Can you work these out from the model? Positions are in its coordinate system, mm. Face numbers are marked on the shaded views. A direction names the side the tool comes from. Give positions to 0.01 mm unless a question says otherwise; leave off trailing zeros. Write each loop counter-clockwise with the first axis right and the second up, starting at its lowest first coordinate (ties: lowest second). Pieces come first, ordered by that corner, then holes. Notation, with made-up numbers: M -26,-4 L 27,-4 A21 cw 27,28 Z; hole C 76,39 d3. An arc over 180 degrees is marked long. Use CSV: the item, a comma, the result in double quotes. Start each with the question number.
from build123d import *

# Parameters (mm, degrees)
F1_DEPTH  = 50.8
F3_DEPTH  = 16.51
F6_DEPTH  = 12.7
F4_R      = 7.62
F7_DEPTH  = 19.05
F8_R      = 6.35
F9_DEPTH  = 70.358
F10_R     = 7.62
F11_DEPTH = 17.018


with BuildPart() as f1:
    # F0 (on Front) → F1 (new body)
    with BuildSketch(Plane.XZ):
        Polygon((-5.651368, 9.435547), (-10.997107, -0.176455), (-5.345739, -9.612001), (5.651368, -9.435547), (10.997107, 0.176455), (5.345739, 9.612001), align=None)
    extrude(amount=F1_DEPTH)

    # F2 (on Right) → F3 (join)
    with BuildSketch(Plane.YZ):
        Polygon((-19.900739, 9.525), (-30.899261, 9.525), (-36.398523, 0), (-30.899261, -9.525), (-19.900739, -9.525), (-14.401477, 0), align=None)
    extrude(amount=-F3_DEPTH)

    # F5 (on face) → F6 (join)
    with BuildSketch(Plane.XZ.offset(50.8)):
        Polygon((-4.356068, 11.679071), (-12.292406, 2.06707), (-7.936338, -9.612001), (4.356068, -11.679071), (12.292406, -2.06707), (7.936338, 9.612001), align=None)
    extrude(amount=F6_DEPTH)

    # F4 (on face) → F7 (join)
    with BuildSketch(Plane(origin=(0, 0, 0), x_dir=(-1, 0, 0), z_dir=(0, 1, 0))):
        Circle(F4_R)
    extrude(amount=F7_DEPTH)

    # F8 (on face) → F9 (cut)
    with BuildSketch(Plane(origin=(0, 19.05, 0), x_dir=(-1, 0, 0), z_dir=(0, 1, 0))):
        Circle(F8_R)
    extrude(amount=-F9_DEPTH, mode=Mode.SUBTRACT)

    # F10 (on face) → F11 (cut)
    with BuildSketch(Plane(origin=(-16.51, 0, 0), x_dir=(0, -1, 0), z_dir=(-1, 0, 0))):
        with Locations((25.4, 0)):
            Circle(F10_R)
    extrude(amount=-F11_DEPTH, mode=Mode.SUBTRACT)


solid = f1.part
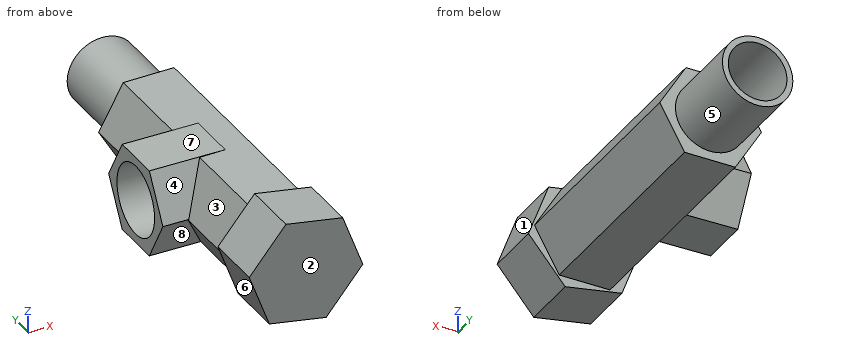
(1) Please list where these lines run through material, in increasing order: L1, parallel to Y at x = -10.75, z = 0; L2, parallel to Z at x = 0, y = -4.5; L3, parallel to Z at x = -9.5, y = -25.4 (3 decimals). Write a range as [from, to].
(2) I want a section at A-A (y = 4.5). Write out the boundary of the cut face in (x, z).
(3) Thinking about a two-plate mould opening in Y: for the marked faces 1, 2 and 3, which applies, released by +Y, released by -Y, zero draft, split by the parting line, or undercut?
(4) Which directions (+Z, -Z, +X, -X, +Y, -Y) give clear straight access to the entire face, cutting with the end or side of a thin tool? Please do the marked faces 4, 5, 6, 7 and 8.
(5) Will these pins go through, and if not, where does the flat tip stop? pin 1 Ø7 at (x, z) = (-1.5, 5.5) entering from +Y; pin 2 Ø10 at (x, y) = (-10.5, -33.5) entering from -Z (3 decimals); pin 3 Ø1.5 at (x, y) = (-3.5, 8.5) entering from -Z; pin 4 Ø8 at (y, z) = (-45, 9) entering from +X.
(6) I want a section at D-D (y = -25.4). Write out the boundary of the cut face in (x, z) (3 decimals), and give its area (3 significant figures).
(7) I want a section at C-C (x = -3.25). Write out the boundary of the cut face in (y, z) (3 decimals), and give its area (3 significant figures).
(8) I want a section at B-B (z = 3.5). Write out the boundary of the cut face in (x, y), and give its area (3 significant figures).
Geometry results:
1,L1,"y = [-63.5, -33.02], [-17.78, 0]"
1,L2,"z = [-9.53, -6.35], [6.35, 9.53]"
1,L3,"z = [-9.525, -7.62], [7.62, 9.525]"
2,outline,"C 0,0 d15.24; hole C 0,0 d12.7"
3,face 1,"zero draft"
3,face 2,"released by -Y"
3,face 3,"undercut"
4,face 4,"+Z, -X"
4,face 5,"+Y"
4,face 6,"-Z, -X, -Y"
4,face 7,"+Z, -X, +Y"
4,face 8,"-Z, -X"
5,pin 1,"stops at y = 19.05"
5,pin 2,"stops at z = -9.525"
5,pin 3,"stops at z = -7.11"
5,pin 4,"stops at x = 8.11"
6,outline,"M -16.51,-9.525 L -5.398,-9.525 L -5.346,-9.612 L 5.651,-9.436 L 10.997,0.176 L 5.346,9.612 L -0.076,9.525 L -16.51,9.525 L -16.51,7.62 L 0.508,7.62 L 0.508,6.33 A6.35 cw 0.508,-6.33 L 0.508,-7.62 L -16.51,-7.62 Z"
6,area,"156 mm2"
7,outline,"M -63.5,-10.4 L -50.8,-10.4 L -50.8,-9.578 L 0,-9.578 L 0,-6.892 L 19.05,-6.892 L 19.05,-5.455 L -20.08,-5.455 A7.62 cw -30.72,-5.455 L -51.308,-5.455 L -51.308,5.455 L -30.72,5.455 A7.62 cw -20.08,5.455 L 19.05,5.455 L 19.05,6.892 L 0,6.892 L 0,9.474 L -19.871,9.474 L -19.901,9.525 L -30.899,9.525 L -30.929,9.474 L -50.8,9.474 L -50.8,11.493 L -63.5,11.493 Z"
7,area,"710 mm2"
8,outline,"M -16.51,-34.38 L -8.95,-34.38 L -8.95,-50.8 L -11.11,-50.8 L -11.11,-63.5 L 10.22,-63.5 L 10.22,-50.8 L 9.01,-50.8 L 9.01,0 L 6.77,0 L 6.77,19.05 L 5.3,19.05 L 5.3,-51.31 L -5.3,-51.31 L -5.3,-32.17 L -16.51,-32.17 Z; M -16.51,-18.63 L -5.3,-18.63 L -5.3,19.05 L -6.77,19.05 L -6.77,0 L -8.95,0 L -8.95,-16.42 L -16.51,-16.42 Z"
8,area,"679 mm2"
